Work out the finished part from the listing and answer in its coordinate system (mm). A direction names the side the tool comes from. Coordinates: 2 decimals unless noted, no trailing zeros. Loops run counter-clockwise (first coordinate to the right, second up) from the corner with the lowest first, then second, coordinate; pieces in that order, holes last. Notation, with made-up numbers: (13, -36.5) -> (67, -36.5) arc R17 cw to (67, -15.5) -> close; hole circle Ø11 at (24, 38). An arc over 180 degrees is marked (long way). Answer as CSV lines item,"result".
```python
from build123d import *

# Parameters (mm, degrees)
F1_DEPTH     = 35
F2_T1_DEPTH  = 30.7885359973
F2_T4_ANGLE  = 105.523431357
F2_T6_ANGLE  = 105.523431357
F2_T8_ANGLE  = 105.523431357
F2_T10_ANGLE = 105.523431357


# Not quite as in the source:
# - a fillet or chamfer that OpenCascade refuses, or shapes differently, is made with other operations: its cross-section is extruded or revolved along the edge and cut away or added


with BuildPart() as f1:
    # F0 (on Front) → F1 (new body)
    with BuildSketch(Plane.XZ):
        with BuildLine():
            ThreePointArc((-8, -10.8742815855), (0, 13.5), (8, -10.8742815855))
            Line((8, -10.8742815855), (8, -12.6885775404))
            ThreePointArc((8, -12.6885775404), (13.1339255366, -7.2456883731), (15, 0))
            Line((15, 0), (15, 18.2885359973))
            Line((15, 18.2885359973), (-15, 18.2885359973))
            Line((-15, 18.2885359973), (-15, 0))
            ThreePointArc((-15, 0), (-13.1339255366, -7.2456883731), (-8, -12.6885775404))
            Line((-8, -12.6885775404), (-8, -10.8742815855))
        make_face()
    extrude(amount=F1_DEPTH)

    # F2: fillet of radius 5 on 4 edges, made by hand

    # F2_s2 → F2_t1 (cut)
    with BuildSketch(Plane.XY):
        with BuildLine():
            ThreePointArc((15, -30), (13.5355339059, -33.5355339059), (10, -35))
            Line((10, -35), (15, -35))
            Line((15, -35), (15, -30))
        make_face()
        with BuildLine():
            ThreePointArc((-15, -30), (-13.5355339059, -33.5355339059), (-10, -35))
            Line((-10, -35), (-15, -35))
            Line((-15, -35), (-15, -30))
        make_face()
        with BuildLine():
            ThreePointArc((15, -5), (13.5355339059, -1.4644660941), (10, 0))
            Line((10, 0), (15, 0))
            Line((15, 0), (15, -5))
        make_face()
        with BuildLine():
            ThreePointArc((-15, -5), (-13.5355339059, -1.4644660941), (-10, 0))
            Line((-10, 0), (-15, 0))
            Line((-15, 0), (-15, -5))
        make_face()
    extrude(amount=F2_T1_DEPTH, mode=Mode.SUBTRACT)

    # F2_s3 → F2_t4 (revolve, cut)
    with BuildSketch(Plane.XY):
        with BuildLine():
            ThreePointArc((-15, -5), (-13.5355339059, -1.4644660941), (-10, 0))
            Line((-10, 0), (-15, 0))
            Line((-15, 0), (-15, -5))
        make_face()
    revolve(axis=Axis((0, 0, 0), (0, -1, 0)), revolution_arc=F2_T4_ANGLE, mode=Mode.SUBTRACT)

    # F2_s5 → F2_t6 (revolve, cut)
    with BuildSketch(Plane(origin=(0, 0, 0), x_dir=(0, 1, 0), z_dir=(-0.9635210843, 0, 0.2676324346))):
        with BuildLine():
            ThreePointArc((-5, 15), (-1.4644660941, 13.5355339059), (0, 10))
            Line((0, 10), (0, 15))
            Line((0, 15), (-5, 15))
        make_face()
    revolve(axis=Axis((0, 0, 0), (0, -1, 0)), revolution_arc=F2_T6_ANGLE, mode=Mode.SUBTRACT)

    # F2_s7 → F2_t8 (revolve, cut)
    with BuildSketch(Plane.XY):
        with BuildLine():
            ThreePointArc((-15, -30), (-13.5355339059, -33.5355339059), (-10, -35))
            Line((-10, -35), (-15, -35))
            Line((-15, -35), (-15, -30))
        make_face()
    revolve(axis=Axis((0, -35, 0), (0, -1, 0)), revolution_arc=F2_T8_ANGLE, mode=Mode.SUBTRACT)

    # F2_s9 → F2_t10 (revolve, cut)
    with BuildSketch(Plane(origin=(0, 0, 0), x_dir=(0, 1, 0), z_dir=(-0.9635210843, 0, 0.2676324346))):
        with BuildLine():
            ThreePointArc((-30, 15), (-33.5355339059, 13.5355339059), (-35, 10))
            Line((-35, 10), (-35, 15))
            Line((-35, 15), (-30, 15))
        make_face()
    revolve(axis=Axis((0, -35, 0), (0, -1, 0)), revolution_arc=F2_T10_ANGLE, mode=Mode.SUBTRACT)


solid = f1.part
```
(1) A cutting plane is placed at C-C, the plane z = 3.5. Write down the section's boundary in (x, y), and give its area (3 significant figures).
Computed values:
outline,"(-15, -30) arc R5 ccw to (-13.04, -33.97) -> (-13.04, -1.03) arc R5 ccw to (-15, -5) -> close; (13.04, -33.97) arc R5 ccw to (15, -30) -> (15, -5) arc R5 ccw to (13.04, -1.03) -> close"
area,"120 mm2"
(2) For a pull along Z with two mould halves and no side action, classify faces 1 (the face through (8, -17, -12)), 2 (the face through (-0.47, -17.26, 13.49)), 3 (the face through (-13.185, -17.325, -7.153)) as pulls with the +Z half, pulls with the -Z half, needs draft (parallel to the pull), parting line crosses it, or undercut.
Computed values:
face 1,"needs draft"
face 2,"undercut"
face 3,"pulls with the -Z half"
(3) Consider line 1 along X through (y, z) = (-27.5, 0); line 2 along Z through (x, y) = (-11.5, -18); line 3 along Z through (x, y) = (-8.5, -19.5). Determine where each line is inside the solid, lowest interval first.
Computed values:
line 1,"-15 to -13.5, 13.5 to 15"
line 2,"-9.63 to -7.07, 7.07 to 18.29"
line 3,"-12.36 to -10.49, 10.49 to 18.29"
(4) A cutting plane is placed at D-D, the plane x = 0. Write down the section's boundary in (y, z), and give its area (3 significant figures).
Computed values:
outline,"(-35, 13.5) -> (0, 13.5) -> (0, 18.29) -> (-35, 18.29) -> close"
area,"168 mm2"
(5) A cutting plane is placed at A-A, the plane z = 15.5. Write down the section's boundary in (x, y).
Computed values:
outline,"(-15, -30) arc R5 ccw to (-10, -35) -> (10, -35) arc R5 ccw to (15, -30) -> (15, -5) arc R5 ccw to (10, 0) -> (-10, 0) arc R5 ccw to (-15, -5) -> close"
(6) Flat-ended cylindrical pins translate along their axes: pin 1 Ø2 at (y, z) = (-19.5, -11.5) entering from -X; pin 2 Ø8 at (x, z) = (-0.5, 8) entering from +Y; pin 3 Ø4 at (y, z) = (-19, -4) entering from +X; pin 4 Ø0.5 at (y, z) = (-22, -12) entering from +X. Find the tip coordinate at first contact, or state that the pin passes through.
Computed values:
pin 1,"x = -10.71"
pin 2,"through"
pin 3,"x = 14.87"
pin 4,"x = 9.32"
(7) A cutting plane is placed at B-B, the plane y = -7.5. Write down the section's boundary in (x, z).
Computed values:
outline,"(-15, 0) arc R15 ccw to (-8, -12.69) -> (-8, -10.87) arc R13.5 cw (long way) to (8, -10.87) -> (8, -12.69) arc R15 ccw to (15, 0) -> (15, 18.29) -> (-15, 18.29) -> close"
(8) Which of the six approach directions +Z, -Z, +X, -X, +Y, -Y give full straight-line access (tool end or side, diameter ignored) to faces 4 (the face through (0, 0, 15)), 5 (the face through (-8, -17, -12))?
Computed values:
face 4,"+Z, -Z, +X, -X, +Y"
face 5,"-Z, +Y, -Y"
